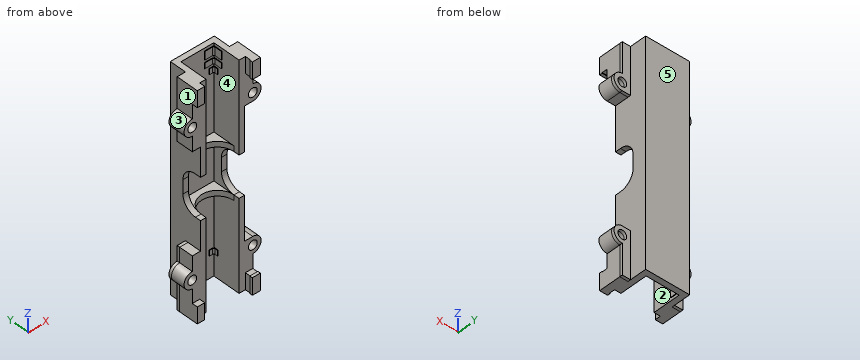
```python
from build123d import *

# Parameters (mm, degrees)
BOSS_EXTRUDE1_DEPTH      = 34.25
BOSS_EXTRUDE2_DEPTH      = 6.2
BOSS_EXTRUDE3_DEPTH      = 6.2
SKETCH9_R                = 1.6
BOSS_EXTRUDE4_DEPTH      = 5
CUT_EXTRUDE1_START       = -16
SKETCH10_W               = 15
SKETCH10_H               = 7
CUT_EXTRUDE1_DEPTH       = 16
SKETCH11_W               = 12
SKETCH11_H               = 2
BOSS_EXTRUDE5_DEPTH      = 2
FILLET1_R                = 6
BOSS_EXTRUDE6_DEPTH      = 3
BOSS_EXTRUDE7_DEPTH      = 2
BOSS_EXTRUDE8_DEPTH      = 2
CIRPATTERN1_COUNT        = 2
FILLET2_R                = 0.5
FILLET4_R                = 5
BOSS_EXTRUDE9_DEPTH      = 6.1
BOSS_EXTRUDE10_START     = -5
BOSS_EXTRUDE10_OUTLINE_W = 3
BOSS_EXTRUDE10_OUTLINE_H = 4.9
BOSS_EXTRUDE10_DEPTH     = 5
SKETCH17_W               = 3
SKETCH17_H               = 4.9
BOSS_EXTRUDE11_DEPTH     = 5
BOSS_EXTRUDE12_START     = -5
BOSS_EXTRUDE12_OUTLINE_W = 3
BOSS_EXTRUDE12_OUTLINE_H = 5.4
BOSS_EXTRUDE12_DEPTH     = 5
CUT_EXTRUDE2_DEPTH       = 2
SKETCH21_R               = 1.6
BOSS_EXTRUDE13_DEPTH     = 1


# Read off the part's stored shape, not the designer's step: Boss-Extrude10, Boss-Extrude12
# Some blends are built 0.0001 mm under size
with BuildPart() as part:
    # Sketch1 → Boss-Extrude1 (new, symmetric)
    with BuildSketch(Plane.XY):
        Polygon((-8, -5), (-8, 7), (8, 7), (8, -5), (6, -5), (6, 5), (-6, 5), (-6, -5), align=None)
    extrude(amount=BOSS_EXTRUDE1_DEPTH, both=True)

    # Sketch6 → Boss-Extrude2 (add)
    with BuildSketch(Plane.XY.offset(34.25)):
        Polygon((6, 5), (6, -5), (8, -5), (8, 7), (-8, 7), (-8, -5), (-6, -5), (-6, 5), align=None)
    extrude(amount=BOSS_EXTRUDE2_DEPTH)

    # Sketch8 → Boss-Extrude3 (add)
    with BuildSketch(Plane(origin=(0, 0, -34.25), x_dir=(-1, 0, 0), z_dir=(0, 0, -1))):
        Polygon((-6, -5), (-6, 5), (6, 5), (6, -5), (8, -5), (8, 7), (-8, 7), (-8, -5), align=None)
    extrude(amount=BOSS_EXTRUDE3_DEPTH)

    # Sketch9 → Boss-Extrude4 (add)
    # profile 1 of 4: a face of its own
    with BuildSketch(Plane.XZ.offset(5)):
        with BuildLine():
            Line((-11, 29.45), (-6, 29.45))
            Line((-6, 29.45), (-6, 23.45))
            Line((-6, 23.45), (-11, 23.45))
            ThreePointArc((-11, 23.45), (-14, 26.45), (-11, 29.45))
        make_face()
        with Locations(Location((-11, 26.45, 0), (0, 0, 270))):
            Circle(SKETCH9_R, mode=Mode.SUBTRACT)
    # profile 2 of 4: a face of its own
    with BuildSketch(Plane.XZ.offset(5)):
        with BuildLine():
            Line((11, 29.45), (6, 29.45))
            Line((6, 29.45), (6, 23.45))
            Line((6, 23.45), (11, 23.45))
            ThreePointArc((11, 23.45), (14, 26.45), (11, 29.45))
        make_face()
        with Locations(Location((11, 26.45, 0), (0, 0, 270))):
            Circle(SKETCH9_R, mode=Mode.SUBTRACT)
    # profile 3 of 4: a face of its own
    with BuildSketch(Plane.XZ.offset(5)):
        with BuildLine():
            Line((6, -23.45), (11, -23.45))
            ThreePointArc((11, -23.45), (14, -26.45), (11, -29.45))
            Line((11, -29.45), (6, -29.45))
            Line((6, -29.45), (6, -23.45))
        make_face()
        with Locations(Location((11, -26.45, 0), (0, 0, 90))):
            Circle(SKETCH9_R, mode=Mode.SUBTRACT)
    # profile 4 of 4: a face of its own
    with BuildSketch(Plane.XZ.offset(5)):
        with BuildLine():
            Line((-6, -23.45), (-11, -23.45))
            ThreePointArc((-11, -23.45), (-14, -26.45), (-11, -29.45))
            Line((-11, -29.45), (-6, -29.45))
            Line((-6, -29.45), (-6, -23.45))
        make_face()
        with Locations(Location((-11, -26.45, 0), (0, 0, 90))):
            Circle(SKETCH9_R, mode=Mode.SUBTRACT)
    extrude(amount=-BOSS_EXTRUDE4_DEPTH)

    # Sketch10 → Cut-Extrude1 (cut)
    with BuildSketch(Plane.ZY.offset(8).offset(CUT_EXTRUDE1_START)):
        with Locations((0, -1.5)):
            Rectangle(SKETCH10_W, SKETCH10_H)
    extrude(amount=CUT_EXTRUDE1_DEPTH, mode=Mode.SUBTRACT)

    # Sketch11 → Boss-Extrude5 (add)
    with BuildSketch(Plane(origin=(0, 0, 7.5), x_dir=(-1, 0, 0), z_dir=(0, 0, -1))):
        with Locations((0, 4)):
            Rectangle(SKETCH11_W, SKETCH11_H)
    boss_extrude5 = extrude(amount=-BOSS_EXTRUDE5_DEPTH)

    # Mirror1: Boss-Extrude5 across plane
    add(boss_extrude5.mirror(Plane.XY))

    # Fillet1
    # the kernel refuses this fillet: 6 mm, written as the material it adds along each edge
    with BuildSketch(Plane(origin=(-6, 3, -7.5), x_dir=(0, -1, 0), z_dir=(0, 0, -1)), Plane(origin=(6, 3, 7.5), x_dir=(0, -1, 0), z_dir=(0, 0, 1))) as fillet1_piece_1:
        with BuildLine():
            CenterArc((FILLET1_R, -FILLET1_R), FILLET1_R, 90, 90)
            Line((0, -FILLET1_R), (0, 0))
            Line((0, 0), (FILLET1_R, 0))
        make_face()
    extrude(amount=2)
    with BuildSketch(Plane(origin=(6, 3, -7.5), x_dir=(0, -1, 0), z_dir=(0, 0, -1)), Plane(origin=(-6, 3, 7.5), x_dir=(0, -1, 0), z_dir=(0, 0, 1))) as fillet1_piece_2:
        with BuildLine():
            CenterArc((FILLET1_R, FILLET1_R), FILLET1_R, 180, 90)
            Line((0, FILLET1_R), (0, 0))
            Line((0, 0), (FILLET1_R, 0))
        make_face()
    extrude(amount=2)

    # Sketch12 → Boss-Extrude6 (add)
    with BuildSketch(Plane.XY.offset(39.45)):
        Polygon((2.5, 5), (2.5, 4.8), (5.8, 4.8), (5.8, 1.8), (6, 1.8), (6, 5), align=None)
    boss_extrude6 = extrude(amount=-BOSS_EXTRUDE6_DEPTH)

    # Sketch13 → Boss-Extrude7 (add)
    with BuildSketch(Plane(origin=(0, 0, 35.45), x_dir=(-1, 0, 0), z_dir=(0, 0, -1))):
        Polygon((-2.5, 5), (-6, 5), (-6, 1.8), (-5.8, 1.8), (-5.8, 4.8), (-2.5, 4.8), align=None)
    boss_extrude7 = extrude(amount=BOSS_EXTRUDE7_DEPTH)

    # Sketch14 → Boss-Extrude8 (add)
    with BuildSketch(Plane(origin=(0, 0, 32.45), x_dir=(-1, 0, 0), z_dir=(0, 0, -1))):
        Polygon((-6, 5), (-4.25, 5), (-4.25, 4.8), (-5.8, 4.8), (-5.8, 3.4), (-6, 3.4), align=None)
        Polygon((5.8, 3.4), (5.8, 4.8), (4.25, 4.8), (4.25, 5), (6, 5), (6, 3.4), align=None)
    boss_extrude8 = extrude(amount=BOSS_EXTRUDE8_DEPTH)

    # CirPattern1: Boss-Extrude6, Boss-Extrude7, Boss-Extrude8 ×2 about axis
    cirpattern1_axis = Axis((0, 0, 0), (0, 1, 0))
    add([boss_extrude6.rotate(cirpattern1_axis, i * 360 / CIRPATTERN1_COUNT) for i in range(1, CIRPATTERN1_COUNT)])
    add([boss_extrude7.rotate(cirpattern1_axis, i * 360 / CIRPATTERN1_COUNT) for i in range(1, CIRPATTERN1_COUNT)])
    add([boss_extrude8.rotate(cirpattern1_axis, i * 360 / CIRPATTERN1_COUNT) for i in range(1, CIRPATTERN1_COUNT)])

    # Fillet2
    fillet2_edges = [part.edges().sort_by_distance(p)[0] for p in [
        (5.8, 4.8, 37.95),
        (5.8, 4.8, 34.45),
        (5.8, 4.8, 31.45),
        (-5.8, 4.8, 31.45),
        (-5.8, 4.8, -37.95),
        (-5.8, 4.8, -34.45),
        (-5.8, 4.8, -31.45),
        (5.8, 4.8, -31.45),
    ]]
    fillet(fillet2_edges, radius=FILLET2_R)

    # Fillet4
    fillet4_edges = [part.edges().sort_by_distance(p)[0] for p in [
        (7, 2, -7.5),
        (-7, 2, -7.5),
        (7, 2, 7.5),
        (-7, 2, 7.5),
    ]]
    fillet(fillet4_edges, radius=FILLET4_R - 0.0001)  # a hair under: the kernel refuses the full size

    # Sketch15 → Boss-Extrude9 (add)
    with BuildSketch(Plane.XY.offset(40.45)):
        Polygon((8, -5), (8.1, -5), (8.1, -8), (11, -8), (11, 0), (8, 0), align=None)
        Polygon((-8, -5), (-8.1, -5), (-8.1, -7), (-11, -7), (-11, 0), (-8, 0), align=None)
    boss_extrude9 = extrude(amount=-BOSS_EXTRUDE9_DEPTH)

    # Boss-Extrude10 outline → Boss-Extrude10 (add)
    with BuildSketch(Plane(origin=(0, 0, 0), x_dir=(1, 0, 0), z_dir=(0, 1, 0)).offset(BOSS_EXTRUDE10_START)):
        with Locations((9.5, -31.9)):
            Rectangle(BOSS_EXTRUDE10_OUTLINE_W, BOSS_EXTRUDE10_OUTLINE_H)
        with Locations((-9.5, -31.9)):
            Rectangle(BOSS_EXTRUDE10_OUTLINE_W, BOSS_EXTRUDE10_OUTLINE_H)
    extrude(amount=BOSS_EXTRUDE10_DEPTH)

    # Mirror3: Boss-Extrude9 across plane
    add(boss_extrude9.mirror(Plane.XY))

    # Sketch17 → Boss-Extrude11 (add)
    with BuildSketch(Plane(origin=(0, 0, 0), x_dir=(1, 0, 0), z_dir=(0, 1, 0))):
        with Locations((-9.5, 31.9)):
            Rectangle(SKETCH17_W, SKETCH17_H)
        with Locations((9.5, 31.9)):
            Rectangle(SKETCH17_W, SKETCH17_H)
    extrude(amount=-BOSS_EXTRUDE11_DEPTH)

    # Boss-Extrude12 outline → Boss-Extrude12 (add)
    with BuildSketch(Plane.XZ.offset(5).offset(BOSS_EXTRUDE12_START)):
        with Locations((-9.5, -20.75)):
            Rectangle(BOSS_EXTRUDE12_OUTLINE_W, BOSS_EXTRUDE12_OUTLINE_H)
        with Locations((-9.5, 20.75)):
            Rectangle(BOSS_EXTRUDE12_OUTLINE_W, BOSS_EXTRUDE12_OUTLINE_H)
    extrude(amount=BOSS_EXTRUDE12_DEPTH)

    # Sketch20 → Cut-Extrude2 (cut)
    with BuildSketch(Plane.XZ.offset(7)):
        Polygon((-8.3, -34.35), (-11, -34.35), (-11, -34.55), (-8.3, -34.55), (-8.3, -40.45), (-8.1, -40.45), (-8.1, -34.55), (-8.1, -34.35), align=None)
        Polygon((8.3, 40.45), (8.1, 40.45), (8.1, 34.55), (8.1, 34.35), (8.3, 34.35), (11, 34.35), (11, 34.55), (8.3, 34.55), align=None)
        Polygon((8.1, -34.35), (11, -34.35), (11, -34.55), (8.3, -34.55), (8.3, -40.45), (8.1, -40.45), align=None)
        Polygon((-11, 34.35), (-8.1, 34.35), (-8.1, 40.45), (-8.3, 40.45), (-8.3, 34.55), (-11, 34.55), align=None)
    extrude(amount=-CUT_EXTRUDE2_DEPTH, mode=Mode.SUBTRACT)

    # Sketch21 → Boss-Extrude13 (add)
    # profile 1 of 4: a face of its own
    with BuildSketch(Plane(origin=(0, 0, 0), x_dir=(1, 0, 0), z_dir=(0, 1, 0))):
        with BuildLine():
            Line((-11, -29.45), (-11, -40.45))
            Line((-11, -40.45), (-8, -40.45))
            Line((-8, -40.45), (-8, -18.05))
            Line((-8, -18.05), (-11, -18.05))
            Line((-11, -18.05), (-11, -23.45))
            ThreePointArc((-11, -23.45), (-14, -26.45), (-11, -29.45))
        make_face()
        with Locations(Location((-11, -26.45, 0), (0, 0, 90))):
            Circle(SKETCH21_R, mode=Mode.SUBTRACT)
    # profile 2 of 4: a face of its own
    with BuildSketch(Plane(origin=(0, 0, 0), x_dir=(1, 0, 0), z_dir=(0, 1, 0))):
        with BuildLine():
            Line((11, -23.45), (8, -23.45))
            Line((8, -23.45), (8, -40.45))
            Line((8, -40.45), (11, -40.45))
            Line((11, -40.45), (11, -29.45))
            ThreePointArc((11, -29.45), (14, -26.45), (11, -23.45))
        make_face()
        with Locations(Location((11, -26.45, 0), (0, 0, 90))):
            Circle(SKETCH21_R, mode=Mode.SUBTRACT)
    # profile 3 of 4: a face of its own
    with BuildSketch(Plane(origin=(0, 0, 0), x_dir=(1, 0, 0), z_dir=(0, 1, 0))):
        with BuildLine():
            Line((8, 40.45), (8, 23.45))
            Line((8, 23.45), (11, 23.45))
            ThreePointArc((11, 23.45), (14, 26.45), (11, 29.45))
            Line((11, 29.45), (11, 40.45))
            Line((11, 40.45), (8, 40.45))
        make_face()
        with Locations(Location((11, 26.45, 0), (0, 0, 270))):
            Circle(SKETCH21_R, mode=Mode.SUBTRACT)
    # profile 4 of 4: a face of its own
    with BuildSketch(Plane(origin=(0, 0, 0), x_dir=(1, 0, 0), z_dir=(0, 1, 0))):
        with BuildLine():
            Line((-8, 18.05), (-8, 40.45))
            Line((-8, 40.45), (-11, 40.45))
            Line((-11, 40.45), (-11, 29.45))
            ThreePointArc((-11, 29.45), (-14, 26.45), (-11, 23.45))
            Line((-11, 23.45), (-11, 18.05))
            Line((-11, 18.05), (-8, 18.05))
        make_face()
        with Locations(Location((-11, 26.45, 0), (0, 0, 270))):
            Circle(SKETCH21_R, mode=Mode.SUBTRACT)
    extrude(amount=BOSS_EXTRUDE13_DEPTH)


solid = part.part
```
CAD build for the part. Positions are in the model's coordinates, mm. Face numbers are marked on the shaded views. A direction names the side the tool comes from. Coordinates: 2 decimals unless noted, no trailing zeros. Loops run counter-clockwise (first coordinate to the right, second up) from the corner with the lowest first, then second, coordinate; pieces in that order, holes last. Notation, with made-up numbers: (-38, -5) - (14, -5) arc R23 ccw to (14, 9) - close; hole circle Ø5 at (-25, 32.5). An arc over 180 degrees is marked (long way). Return JSON: item names as keys, results as strings.
1. Drop flat-ended pins along their axis: pin 1 (1 mm diameter, centred on y = 4, z = 32, fed in from +X); pin 2 (1 mm diameter, centred on y = 4, z = -31.5, fed in from -X); pin 3 (4 mm diameter, centred on x = -10.5, z = 28.5, fed in from -Y). Give the stop position or say it passes through.
Result:
{"pin 1": "stops at x = 8", "pin 2": "stops at x = -8", "pin 3": "stops at y = -5"}
2. Band-saw the part on A-A (z = -26.45). Give the cut face in (x, y), and give its area (3 significant figures).
Result:
{"outline": "(-14, -5) - (-12.6, -5) - (-12.6, 1) - (-14, 1) - close; (-9.4, -5) - (-6, -5) - (-6, 5) - (6, 5) - (6, -5) - (9.4, -5) - (9.4, 1) - (8, 1) - (8, 7) - (-8, 7) - (-8, 1) - (-9.4, 1) - close; (12.6, -5) - (14, -5) - (14, 1) - (12.6, 1) - close", "area": "106 mm2"}
3. Band-saw the part on C-C (x = -1.5). Give the cut face in (y, z), and give its area (3 significant figures).
Result:
{"outline": "(2.81, -9.5) - (5, -9.5) - (5, -40.45) - (7, -40.45) - (7, 40.45) - (5, 40.45) - (5, 9.5) - (2.81, 9.5) - (2.81, 7.5) - (5, 7.5) - (5, -7.5) - (2.81, -7.5) - close", "area": "171 mm2"}
4. Probe L1, parallel to X at y = -3.3, z = -26.45; L2, parallel to X at y = 0.25, z = -21; L3, parallel to X at y = 3, z = 23.5. List the from-to ranges inside material, lowest first. Write a range as from..to.
Result:
{"L1": "x = -14..-12.6, -9.4..-6, 6..9.4, 12.6..14", "L2": "x = -11..-6, 6..8", "L3": "x = -8..-6, 6..8"}
5. Mould opens along Z. For the marked faces 4 and 5 say: released by +Z, released by -Z, zero draft, split by the parting line, or undercut.
Result:
{"face 4": "undercut", "face 5": "zero draft"}
6. 3-axis set-ups, long thin cutter, end or side, ignore diameter. For the marked faces 1, 2 and 3: which of +Z, -Z, +X, -X, +Y, -Y reach the whole face in a straight line?
Result:
{"face 1": "+Z, -X, +Y, -Y", "face 2": "-Y", "face 3": "-X, +Y, -Y"}
7. Band-saw the part on D-D (y = 5.75). Give the cut face in (x, z).
Result:
{"outline": "(-8, -40.45) - (8, -40.45) - (8, 40.45) - (-8, 40.45) - close"}
8. Band-saw the part on B-B (z = -16.5). Give the cut face in (x, y).
Result:
{"outline": "(-8, -5) - (-6, -5) - (-6, 5) - (6, 5) - (6, -5) - (8, -5) - (8, 7) - (-8, 7) - close"}
